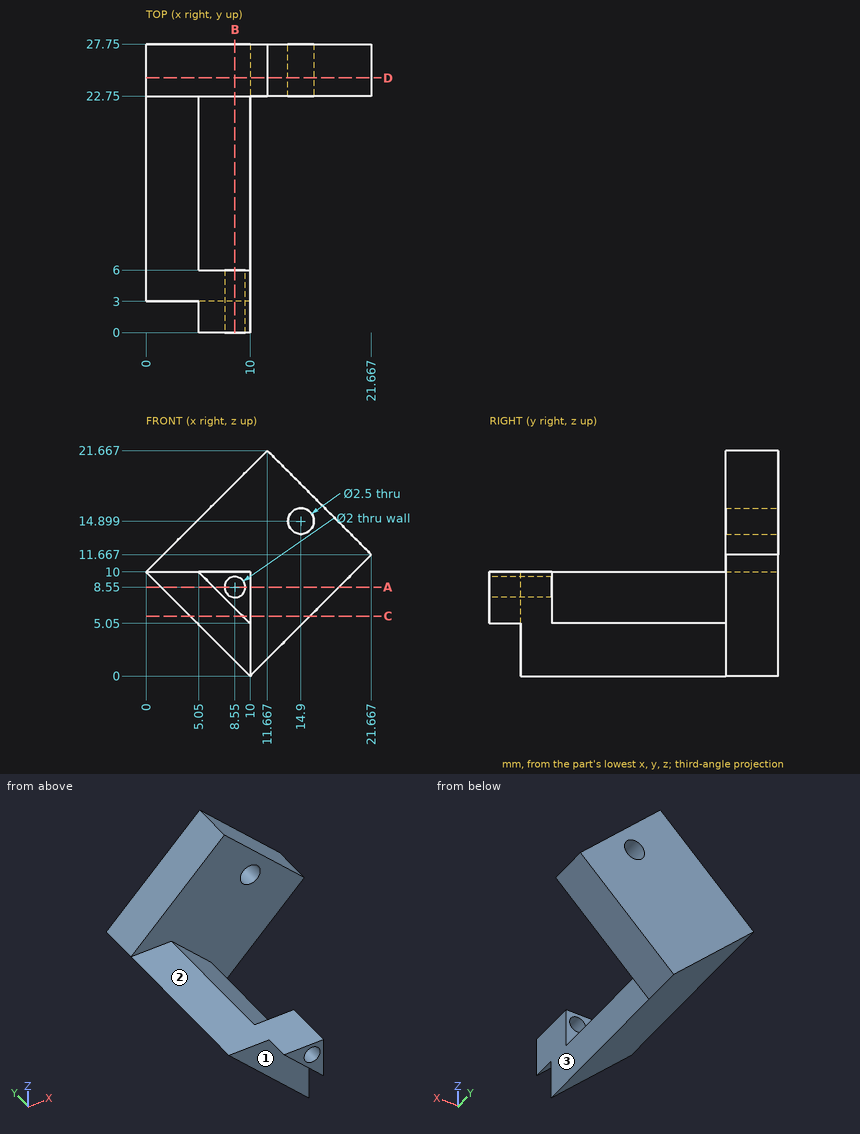
Study the drawing (mm; zero at the part's minimum x, y, z) and answer. A direction names the side the tool comes from. Give positions to 0.01 mm unless a question says otherwise; leave off trailing zeros. Order: outer loops, then holes, each group sorted by start corner. A loop starts at its lowest first (then second) coordinate and runs counter-clockwise, first axis right, second up. Notation, with made-up numbers: (63, 12.5) - (70, 12.5) arc R18 cw to (70, 43.5) - close; hole circle Ø2 at (38, 9). An arc over 180 degrees is marked (long way). Answer in a Markdown table with one row per item. Add a question column.
Q1. The part is cut by section B-B (x = 8.55). Determine the outline of the cut face in (y, z).
Q2. The part is cut by section C-C (z = 5.75). Determine the outline of the cut face in (x, y).
Q3. Find the intervals of material crossed by line 1 along Y through (x, z) = (9, 18.5); line 2 along Y through (x, z) = (8.75, 7.25); line 3 along Z through (x, y) = (8.55, 2.5), in increasing order. Write a range as [from, to].
Q4. The part is cut by section D-D (y = 24.5). Determine the outline of the cut face in (x, z).
Q5. Which of the six approach directions +Z, -Z, +X, -X, +Y, -Y give full straight-line access (tool end or side, diameter ignored) to the marked faces 1, 2 and 3?
Q6. Given P1, Ø11, axis at y = 13, z = 4, coming from the +X side; P2, Ø8, axis at x = 5, y = 13.5, coming from the +Z side; P3, Ø5, axis at x = 5, y = 16, coming from the -Z side; P4, Ø8, axis at x = 6.5, z = 4.5, coming from the -Y side, each flat-ended and moving along its own axis, determine where each tip first touches the part or whether it passes through.
Q7. The part is cut by section A-A (z = 8.55). Determine the outline of the cut face in (x, y).
Determined:
| question | item | result |
|---|---|---|
| 1 | outline | (0, 6.5) - (3, 6.5) - (3, 1.45) - (27.75, 1.45) - (27.75, 18.55) - (22.75, 18.55) - (22.75, 6.5) - (6, 6.5) - (6, 7.55) - (0, 7.55) - close; (0, 9.55) - (6, 9.55) - (6, 10) - (0, 10) - close |
| 2 | outline | (4.25, 3) - (9.3, 3) - (9.3, 0) - (10, 0) - (10, 6) - (9.3, 6) - (9.3, 22.75) - (15.75, 22.75) - (15.75, 27.75) - (4.25, 27.75) - close |
| 3 | line 1 | y = [22.75, 27.75] |
| 3 | line 2 | y = [0, 6], [22.75, 27.75] |
| 3 | line 3 | z = [6.5, 7.55], [9.55, 10] |
| 4 | outline | (0, 10) - (10, 0) - (21.67, 11.67) - (11.67, 21.67) - close; hole circle Ø2.5 at (14.9, 14.9) |
| 5 | face 1 | -Z, -X, -Y |
| 5 | face 2 | +Z, +X, -X, -Y |
| 5 | face 3 | +Z, -Z, +X, -Y |
| 6 | P1 | stops at x = 10 |
| 6 | P2 | stops at z = 10 |
| 6 | P3 | stops at z = 2.5 |
| 6 | P4 | stops at y = 0 |
| 7 | outline | (1.45, 3) - (6.5, 3) - (6.5, 0) - (7.55, 0) - (7.55, 6) - (6.5, 6) - (6.5, 22.75) - (18.55, 22.75) - (18.55, 27.75) - (1.45, 27.75) - close; (9.55, 0) - (10, 0) - (10, 6) - (9.55, 6) - close |
